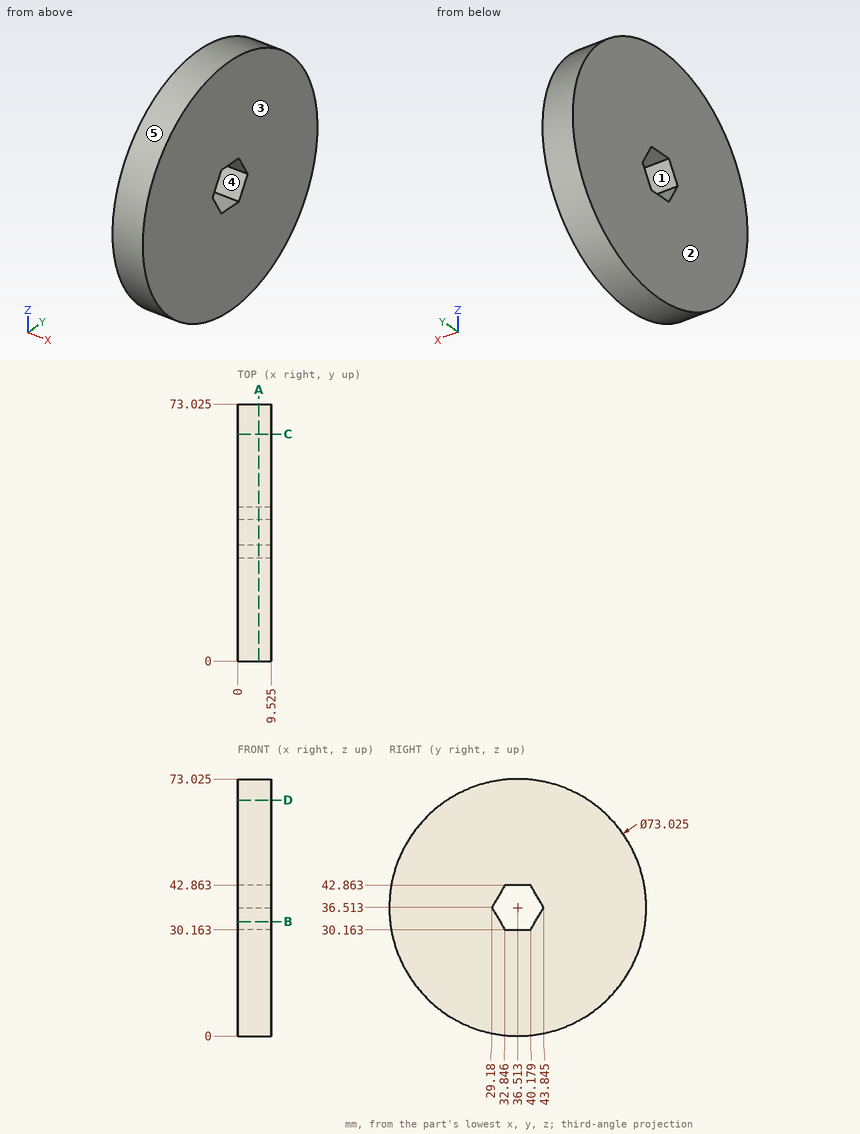
Check sheet for the drawn part. Datum: minimum x, y, z corner. Units: mm. A direction names the side the tool comes from. Round coordinates to 2 decimals unless told otherwise and drop trailing zeros. Loops run counter-clockwise (first coordinate to the right, second up) from the corner with the lowest first, then second, coordinate; pieces in that order, holes last. Notation, with made-up numbers: (33.5, 10) -> (69.5, 10) arc R14 ccw to (69.5, 29) -> close; hole circle Ø7 at (-17, 46.5). An arc over 180 degrees is marked (long way). Put each result on its own line as item: value. Start each with the question number.
1. Section check B-B (z = 32.5). Enter the section's corners in (x, y) (1 decimal).
2. Section check C-C (y = 64.5). Enter the section's corners in (x, z) (1 decimal).
3. Section check D-D (z = 67). Enter the section's corners in (x, y) (1 decimal).
4. Section check A-A (x = 6). Enter the section's corners in (y, z) (1 decimal).
5. Access from +Z, -Z, +X, -X, +Y, -Y to the whole of each face (thin tool, end or side, straight path). Record for the marked faces 1 and 2.
6. Draft check along Y on the marked faces 3, 4 and 5. Enter one of: +Y half, -Y half, draft (parallel to the pull), parting line (faces both ways), or undercut.
7. Scan lines: probe 1 along Y at (x, z) = (1.25, 34.5) (1 decimal); probe 2 along Y at (x, z) = (8.5, 38) (1 decimal); probe 3 along Z at (x, y) = (2, 39) (1 decimal). Record each from-to range of solid material in increasing order.
8. Gauge pin test, flat ends, axial feed: pin 1 (1 mm diameter, centred on x = 4.5, z = 50.5, fed in from +Y); pin 2 (5 mm diameter, centred on x = 3.5, z = 12.5, fed in from -Y); pin 3 (1.5 mm diameter, centred on x = 1, z = 63.5, fed in from +Y) (1 decimal). Record the tip position at first contact, or that the pin passes through.
Findings:
1. outline: (0, 0.2) -> (9.5, 0.2) -> (9.5, 31.5) -> (0, 31.5) -> close; (0, 41.5) -> (9.5, 41.5) -> (9.5, 72.8) -> (0, 72.8) -> close
2. outline: (0, 13.1) -> (9.5, 13.1) -> (9.5, 60) -> (0, 60) -> close
3. outline: (0, 16.4) -> (9.5, 16.4) -> (9.5, 56.6) -> (0, 56.6) -> close
4. outline: circle Ø73 at (36.5, 36.5); hole (29.2, 36.5) -> (32.8, 30.2) -> (40.2, 30.2) -> (43.8, 36.5) -> (40.2, 42.9) -> (32.8, 42.9) -> close
5. face 1: +X, -X
5. face 2: +Z, -Z, -X, +Y, -Y
6. face 3: draft
6. face 4: undercut
6. face 5: parting line
7. probe 1: y = 0.1 to 30.3, 42.7 to 73
7. probe 2: y = 0 to 30, 43 to 73
7. probe 3: z = 0.1 to 30.2, 42.9 to 72.9
8. pin 1: stops at y = 70.44
8. pin 2: stops at y = 7.01
8. pin 3: stops at y = 61.9
